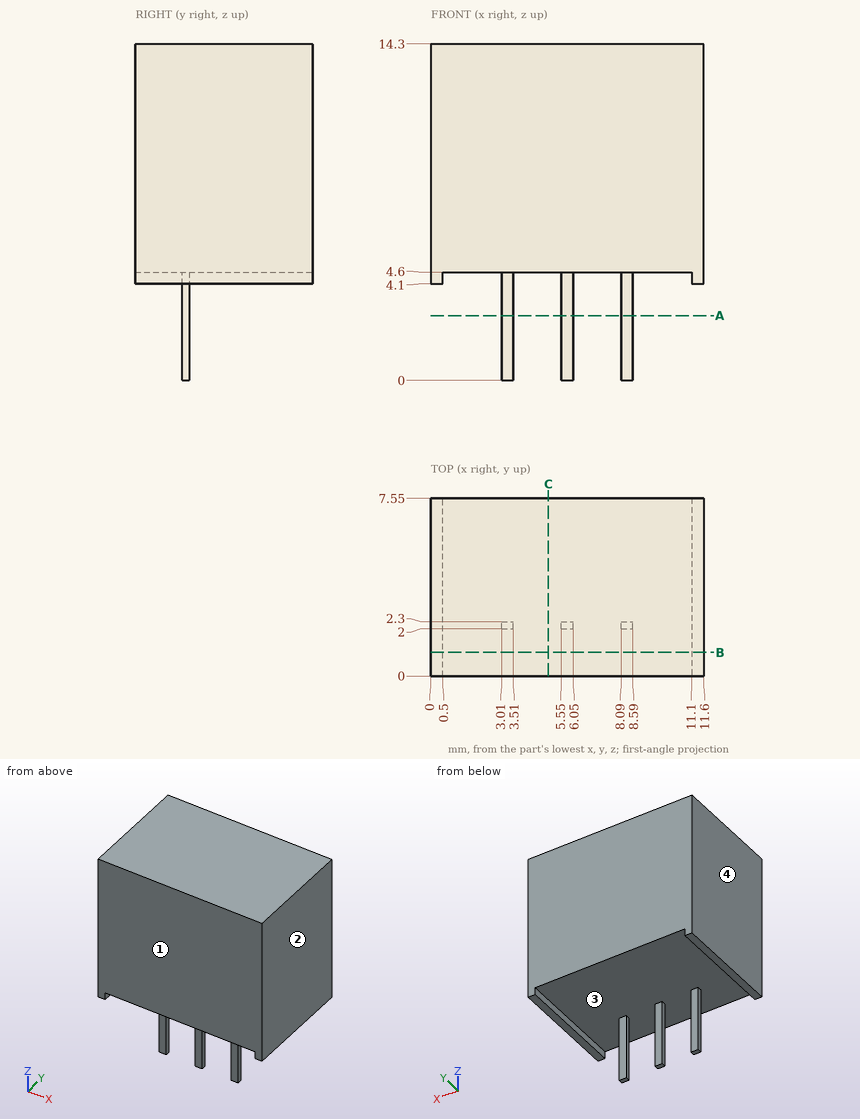
Answer from the drawing. Dimensions are ordinates in mm from the lowest x, y and z of the part. Round coordinates to 2 decimals unless told otherwise and drop trailing zeros. Order: outer loops, then holes, each group sorted by start corner. A loop starts at its lowest first (then second) coordinate and runs counter-clockwise, first axis right, second up. Notation, with made-up numbers: (30, 28.5) - (36, 28.5) arc R21 cw to (36, 55.5) - close; hole circle Ø11 at (35.5, 22). An arc over 180 degrees is marked (long way). Put each result on its own line as item: value. Start each with the question number.
(1) Find section A-A (z = 2.75). Give the vertices of the cut face in (x, y), plus the area to 3 significant figures.
(2) A straight line is drawn through the part: probe 1 along Z at (x, y) = (1.75, 6). Find the intervals that lie inside material, in ascending order. Write a range as from..to.
(3) Determine the mould class of the marked faces 1, 2, 3 and 4 for opening direction X: released by +X, released by -X, zero draft, split by the parting line, or undercut.
(4) Find section B-B (y = 1). Give the vertices of the cut face in (x, z), plus the area to 3 significant figures.
(5) Given P1, Ø0.6, axis at x = 3.5, z = 2, coming from the -Y side; P2, Ø2.5, axis at x = 6.5, y = 3.5, coming from the -Z side, each flat-ended and moving along its own axis, determine where each tip first touches the part or whether it passes through.
(6) Find section C-C (x = 5). Give the vertices of the cut face in (y, z).
Reply:
1. outline: (3.01, 2) - (3.51, 2) - (3.51, 2.3) - (3.01, 2.3) - close; (5.55, 2) - (6.05, 2) - (6.05, 2.3) - (5.55, 2.3) - close; (8.09, 2) - (8.59, 2) - (8.59, 2.3) - (8.09, 2.3) - close
1. area: 0.450 mm^2
2. probe 1: 4.6..14.3
3. face 1: zero draft
3. face 2: released by +X
3. face 3: undercut
3. face 4: released by -X
4. outline: (0, 4.1) - (0.5, 4.1) - (0.5, 4.6) - (11.1, 4.6) - (11.1, 4.1) - (11.6, 4.1) - (11.6, 14.3) - (0, 14.3) - close
4. area: 113 mm^2
5. P1: y = 2
5. P2: z = 4.6
6. outline: (0, 4.6) - (7.55, 4.6) - (7.55, 14.3) - (0, 14.3) - close
